Geometry check sheet. Reference: the model listing, model coordinates, mm. Face numbers are marked on the shaded views. A direction names the side the tool comes from. Round coordinates to 2 decimals unless told otherwise and drop trailing zeros. Write each loop counter-clockwise with the first axis right and the second up, starting at its lowest first coordinate (ties: lowest second). Pieces come first, ordered by that corner, then holes. Notation, with made-up numbers: M 3,73.5 L 52,73.5 A37 ccw 52,110.5 Z; hole C 5,26.5 d6. An arc over 180 degrees is marked long. One line per item, written item: value. Start each with the question number.
1. Section check C-C (y = 0.8). Record the boundary of the cut face in (x, z).
2. Section check A-A (x = 0). Record the boundary of the cut face in (y, z), and give its area (3 significant figures).
3. Access from +Z, -Z, +X, -X, +Y, -Y to the whole of each face (thin tool, end or side, straight path). Record for the marked faces 1 and 2.
4. Depth check by flat-ended pin: P1, Ø0.7, axis at y = 3.5, z = 10, coming from the -X side; P2, Ø1.5, axis at y = 1, z = 10, coming from the +X side; P3, Ø3, axis at x = 0, z = 6.5, coming from the -Y side; P4, Ø0.6, axis at x = 3.5, z = 9, coming from the +Y side. Enter the tip coordinate at first touch or a pass-through.
5. Section check D-D (z = 10). Record the boundary of the cut face in (x, y).
6. Section check B-B (z = 6.5). Record the boundary of the cut face in (x, y), and give its area (3 significant figures).
7. Release check for a two-part mould opening along X. For the marked faces 3, 4, 5 and 6 record: pulls with the +X half, pulls with the -X half, needs draft (parallel to the pull), parting line crosses it, or undercut.
8. Scan lines: probe 1 along Z at (x, y) = (0, 1.65); probe 2 along Z at (x, y) = (-1.75, 0.95); probe 3 along X at (y, z) = (0.7, 12.75). Record each from-to range of solid material in increasing order. Write a range as [from, to].
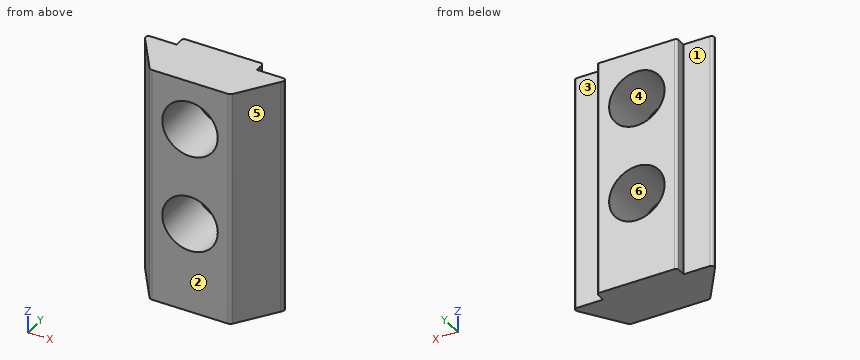
Autodesk Inventor part; units mm, degrees
ref_plane "YZ Plane" through (0, 0, 0) normal (1, 0, 0) x (0, 1, 0)
ref_plane "XZ Plane" through (0, 0, 0) normal (0, 1, 0) x (-1, 0, 0)
ref_plane "XY Plane" through (0, 0, 0) normal (0, 0, 1) x (1, 0, 0)
sketch "Sketch_1" plane through (0, 0, 0) normal (0, 0, 1) x (1, 0, 0)
  arc A0 (-4.7999, 3.3) -> (-4.9858, 3.0264) centre (-4.7999, 3.1) ccw
  arc A1 (-4.9858, 3.0264) -> (-4.8752, 2.8208) centre (-4.056, 3.3944) ccw
  line L0 (-4.8752, 2.8208) -> (-2.9896, 0.1279)
  arc A2 (-2.9896, 0.1279) -> (-2.7438, 0) centre (-2.7438, 0.3) ccw
  line L1 (-2.7438, 0) -> (2.7438, 0)
  arc A3 (2.7438, 0) -> (2.9896, 0.1279) centre (2.7438, 0.3) ccw
  line L2 (2.9896, 0.1279) -> (4.8752, 2.8208)
  arc A4 (4.8752, 2.8208) -> (4.9858, 3.0264) centre (4.056, 3.3944) ccw
  arc A5 (4.9858, 3.0264) -> (4.7999, 3.3) centre (4.7999, 3.1) ccw
  line L3 (4.7999, 3.3) -> (2.9, 3.3)
  line L4 (2.9, 3.3) -> (2.9, 3.9)
  arc A6 (2.9, 3.9) -> (2.7, 4.1) centre (2.7, 3.9) ccw
  line L5 (2.7, 4.1) -> (-2.7, 4.1)
  arc A7 (-2.7, 4.1) -> (-2.9, 3.9) centre (-2.7, 3.9) ccw
  line L6 (-2.9, 3.9) -> (-2.9, 3.3)
  line L7 (-2.9, 3.3) -> (-4.7999, 3.3)
extrude "Extrusion1" add sketch "Sketch_1" along normal blind 17
sketch "Sketch3" plane through (-2.7, 4.1, 0) normal (0, 1, 0) x (1, 0, 0)
  line L0 (0, -17) -> (5.4, -17)
  line L1 (5.4, 0) -> (5.4, -17)
  line L2 (5.4, 0) -> (0, 0)
  circle A0 centre (2.7, -6.5) radius 2
  circle A1 centre (2.7, -13.5) radius 2
  point P0 (2.7, 0)
  dimension "d5" = 4
  dimension "d6" = 6.5
  dimension "d7" = 2.7
  dimension "d8" = 3.5
  dimension "d9" = 4
extrude "Extrusion2" cut sketch "Sketch3" against normal up to next
thread "Thread2"
thread "Thread3"
properties part number "ExtrusionNutLockHNTR5-4"
Result sheet:
1. outline: M -3.46,0 L 3.46,0 L 3.46,17 L -3.46,17 Z; hole C 0,6.5 d4; hole C 0,13.5 d4
2. outline: M 0,0 L 4.1,0 L 4.1,4.5 L 0,4.5 Z; M 0,8.5 L 4.1,8.5 L 4.1,11.5 L 0,11.5 Z; M 0,15.5 L 4.1,15.5 L 4.1,17 L 0,17 Z
2. area: 36.9 mm2
3. face 1: +Z, -Z, -X, +Y
3. face 2: +Z, -Z, +X, -X, -Y
4. P1: stops at x = -4.99
4. P2: stops at x = 4.13
4. P3: passes through
4. P4: stops at y = 3.3
5. outline: M -4.99,3.03 A1.01 ccw -4.88,2.82 L -2.99,0.13 A0.3 ccw -2.74,0 L 2.74,0 A0.3 ccw 2.99,0.13 L 4.88,2.82 A0.99 ccw 4.99,3.03 A0.2 ccw 4.8,3.3 L 2.9,3.3 L 2.9,3.9 A0.2 ccw 2.7,4.1 L -2.7,4.1 A0.2 ccw -2.9,3.9 L -2.9,3.3 L -4.8,3.3 A0.2 ccw Z
6. outline: M -4.99,3.03 A1.01 ccw -4.88,2.82 L -2.99,0.13 A0.3 ccw -2.74,0 L -2,0 L -2,4.1 L -2.7,4.1 A0.2 ccw -2.9,3.9 L -2.9,3.3 L -4.8,3.3 A0.2 ccw Z; M 2,0 L 2.74,0 A0.3 ccw 2.99,0.13 L 4.88,2.82 A0.99 ccw 4.99,3.03 A0.2 ccw 4.8,3.3 L 2.9,3.3 L 2.9,3.9 A0.2 ccw 2.7,4.1 L 2,4.1 Z
6. area: 14.9 mm2
7. face 3: needs draft
7. face 4: undercut
7. face 5: pulls with the +X half
7. face 6: undercut
8. probe 1: z = [0, 4.5], [8.5, 11.5], [15.5, 17]
8. probe 2: z = [0, 5.53], [7.47, 12.53], [14.47, 17]
8. probe 3: x = [-3.39, -1.85], [1.85, 3.39]
